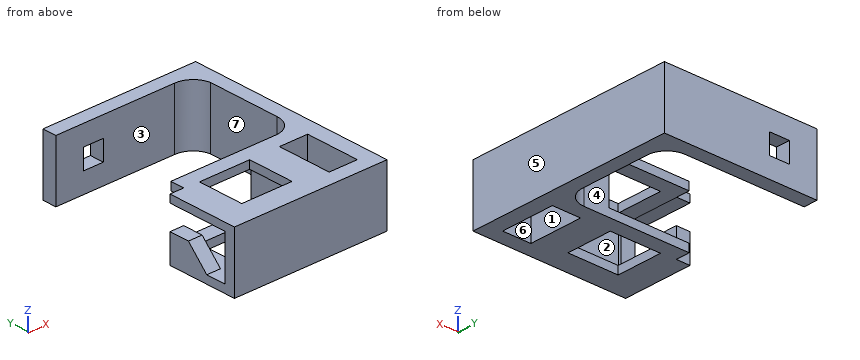
```python
from build123d import *

# Parameters (mm, degrees)
PAD_DEPTH       = 30
POCKET_DEPTH    = 22
POCKET001_DEPTH = 6.9
SKETCH003_W     = 25.3
SKETCH003_H     = 23
SKETCH003_W_2   = 14.2
SKETCH003_H_2   = 27
POCKET002_DEPTH = 30
SKETCH004_W     = 10
SKETCH004_H     = 10
POCKET003_DEPTH = 50


with BuildPart() as part:
    # Sketch → Pad (new body)
    with BuildSketch(Plane.XY):
        with BuildLine():
            Line((-35, 42.015359), (-35, 35.015359))
            Line((-35, 35.015359), (24.9, 35.015359))
            ThreePointArc((34.9, 26.231153), (31.573738, 32.528651), (24.9, 35.015359))
            Line((34.9, -9.768847), (34.9, 26.231153))
            ThreePointArc((24.9, -20), (32.054064, -16.989821), (34.9, -9.768847))
            Line((24.9, -20), (-28.1, -20))
            Line((-28.1, -27), (-28.1, -20))
            Line((-35, -27), (-28.1, -27))
            Line((-35, -27), (-35, -62))
            Line((-35, -62), (41.9, -62))
            Line((41.9, -62), (41.9, 42.015359))
            Line((41.9, 42.015359), (-35, 42.015359))
        make_face()
    extrude(amount=PAD_DEPTH)

    # Sketch001 → Pocket (cut)
    with BuildSketch(Plane.XY.offset(4)):
        Polygon((-28.1, -20), (-28.1, -58.5), (12.2, -58.5), (12.2, -20), (-18.1, -20), (-18.1, -13.5), (-24.1, -13.5), (-24.1, -20), align=None)
    extrude(amount=POCKET_DEPTH, mode=Mode.SUBTRACT)

    # Sketch002 → Pocket001 (cut)
    with BuildSketch(Plane.YZ.offset(-35)):
        Polygon((-27, 26.185834), (-27, 14.185834), (-37, 14.185834), (-47, 4), (-57, 4), (-57, 26.185834), align=None)
    extrude(amount=POCKET001_DEPTH, mode=Mode.SUBTRACT)

    # Sketch003 → Pocket002 (cut)
    with BuildSketch(Plane.XY):
        with Locations((-7.95, -39)):
            Rectangle(SKETCH003_W, SKETCH003_H)
        with Locations((26.8, -41)):
            Rectangle(SKETCH003_W_2, SKETCH003_H_2)
    extrude(amount=POCKET002_DEPTH, mode=Mode.SUBTRACT)

    # Sketch004 → Pocket003 (cut)
    with BuildSketch(Plane.XZ):
        with Locations((-16.1, 15)):
            Rectangle(SKETCH004_W, SKETCH004_H)
    extrude(amount=-POCKET003_DEPTH, mode=Mode.SUBTRACT)


solid = part.part
```
Model file for the job. Use its own axes, mm. Face numbers are marked on the shaded views. A direction names the side the tool comes from. Give positions to 0.01 mm unless a question says otherwise; leave off trailing zeros. Loops run counter-clockwise (first coordinate to the right, second up) from the corner with the lowest first, then second, coordinate; pieces in that order, holes last. Notation, with made-up numbers: (75, 67.25) -> (83, 67.25) arc R22 ccw to (83, 85.25) -> close; hole circle Ø9 at (46.5, -21). An arc over 180 degrees is marked (long way). Write each question's results on one line, items separated by ' | '.
(1) Cut at D-D on x = 22. List the corners of the cut face in (y, z), and give its area (3 significant figures).
Geometry results:
outline: (-62, 0) -> (-54.5, 0) -> (-54.5, 30) -> (-62, 30) -> close; (-27.5, 0) -> (-20, 0) -> (-20, 30) -> (-27.5, 30) -> close; (35.02, 0) -> (42.02, 0) -> (42.02, 30) -> (35.02, 30) -> close | area: 660 mm²
(2) Flat gauge pin, fed straight in: pin 1 Ø1.5 at (y, z) = (11.5, 19.5) entering from -X. Where does the tip first touch, or does it go through?
Geometry results:
pin 1: stops at x = 34.9
(3) Cut at A-A on x = -17. List the corners of the cut face in (y, z), and give its area (3 significant figures).
Geometry results:
outline: (-62, 0) -> (-50.5, 0) -> (-50.5, 4) -> (-58.5, 4) -> (-58.5, 26) -> (-50.5, 26) -> (-50.5, 30) -> (-62, 30) -> close; (-27.5, 0) -> (-20, 0) -> (-20, 4) -> (-27.5, 4) -> close; (-27.5, 26) -> (-20, 26) -> (-20, 30) -> (-27.5, 30) -> close; (35.02, 0) -> (42.02, 0) -> (42.02, 10) -> (35.02, 10) -> close; (35.02, 20) -> (42.02, 20) -> (42.02, 30) -> (35.02, 30) -> close | area: 369 mm²
(4) Cut at B-B on z = 5.5. List the corners of the cut face in (x, y).
Geometry results:
outline: (-35, -62) -> (41.9, -62) -> (41.9, 42.02) -> (-35, 42.02) -> (-35, 35.02) -> (24.9, 35.02) arc R10 cw to (34.9, 26.23) -> (34.9, -9.77) arc R10 cw to (24.9, -20) -> (12.2, -20) -> (12.2, -58.5) -> (-28.1, -58.5) -> (-28.1, -57) -> (-35, -57) -> close; (-35, -45.53) -> (-28.1, -45.53) -> (-28.1, -27) -> (-35, -27) -> close; hole (19.7, -54.5) -> (33.9, -54.5) -> (33.9, -27.5) -> (19.7, -27.5) -> close
(5) Cut at C-C on y = -43.5. List the corners of the cut face in (x, z), and give its area (3 significant figures).
Geometry results:
outline: (-35, 0) -> (-20.6, 0) -> (-20.6, 4) -> (-28.1, 4) -> (-28.1, 7.57) -> (-35, 7.57) -> close; (-35, 26.19) -> (-28.1, 26.19) -> (-28.1, 26) -> (-20.6, 26) -> (-20.6, 30) -> (-35, 30) -> close; (4.7, 0) -> (19.7, 0) -> (19.7, 30) -> (4.7, 30) -> (4.7, 26) -> (12.2, 26) -> (12.2, 4) -> (4.7, 4) -> close; (33.9, 0) -> (41.9, 0) -> (41.9, 30) -> (33.9, 30) -> close | area: 664 mm²
(6) Probe line 1 along Y through (x, z) = (-6, 2.5); line 2 along Y through (x, z) = (21, 8); line 3 along X through (y, z) = (-36, 10). List the from-to ranges inside material, lowest first.
Geometry results:
line 1: y = -62 to -50.5, -27.5 to -20, 35.02 to 42.02 | line 2: y = -62 to -54.5, -27.5 to -20, 35.02 to 42.02 | line 3: x = -35 to -28.1, 12.2 to 19.7, 33.9 to 41.9
(7) Tool access for the marked faces 1, 2 and 3: list every direction of +Z, -Z, +X, -X, +Y, -Y with a clear straight run to the whole face (end or side of a thin tool).
Geometry results:
face 1: +Z, -Z | face 2: none | face 3: +Z, -Z, -X
(8) Pull direction X, two halves, no side cores. Call the marked faces 4, 5, 6 and 7: released by +X, released by -X, zero draft, split by the parting line, or undercut.
Geometry results:
face 4: zero draft | face 5: released by +X | face 6: undercut | face 7: released by -X
